Design review of the part built by this model. Coordinates are the model's own, in mm. Face numbers are marked on the shaded views. A direction names the side the tool comes from. Coordinates: 2 decimals unless noted, no trailing zeros. Write each loop counter-clockwise with the first axis right and the second up, starting at its lowest first coordinate (ties: lowest second). Pieces come first, ordered by that corner, then holes. Notation, with made-up numbers: (31.25, 24.25) -> (47.25, 24.25) arc R32 cw to (47.25, 62.25) -> close; hole circle Ø4 at (66, -30.75). An arc over 180 degrees is marked (long way). Answer in a Markdown table with one row per item. Add a question column.
Item 1: To check wall thickness, follow line 1 (Z direction, x = 0, y = 4); line 2 (X direction, y = 4, z = 2.5). State the ranges of each line that lie inside material, in increasing order.
Item 2: Take a section at B-B, the plane z = 0. Write out the cut boundary in (x, y).
Item 3: For the marked faces 4 and 5, list the 3-axis set-ups (+Z, -Z, +X, -X, +Y, -Y) from which the entire face can be reached by the end or side of a thin tool; tool diameter is ignored.
Item 4: Take a section at A-A, the plane x = 0. Write out the cut boundary in (y, z), and give its area (3 significant figures).
Item 5: Draft analysis for pull direction Z (two halves, no side actions). For the marked faces 1, 2 and 3, state which applies: released by +Z, released by -Z, zero draft, split by the parting line, or undercut.
Item 6: Clearance check with flat-ended pins moving along their axes: P1, Ø0.7, axis at x = 5.5, y = 0.5, coming from the +Z side; P2, Ø1, axis at y = 1.5, z = 5.5, coming from the +X side; P3, Ø0.7, axis at x = -4, y = 0.5, coming from the -Z side. State where each tip first meets the part, or that it passes through.
from build123d import *

# Parameters (mm, degrees)
SKETCH1_R               = 7.9375
SKETCH1_R_2             = 4.25
BOSS_EXTRUDE1_DEPTH     = 6.35
CUT_EXTRUDE1_DEPTH      = 13.896910967
CUT_EXTRUDE1_DEPTH_BACK = 13.896910967
SKETCH2_W               = 7.62
SKETCH2_H               = 2.54
FILLET2_R               = 1.905
FILLET3_R               = 1.27


with BuildPart() as part:
    # Sketch1 → Boss-Extrude1 (new body)
    with BuildSketch(Plane(origin=(0, 0, 0), x_dir=(1, 0, 0), z_dir=(0, 1, 0))):
        with Locations(Location((0, 0, 0), (0, 0, 270))):
            Circle(SKETCH1_R)
        with Locations(Location((0, 0, 0), (0, 0, 270))):
            Circle(SKETCH1_R_2, mode=Mode.SUBTRACT)
    extrude(amount=BOSS_EXTRUDE1_DEPTH)

    # Sketch2 → Cut-Extrude1 (cut, two sides: drawn at the far end of the back side and taken through both)
    with BuildSketch(Plane(origin=(0, 0, 0), x_dir=(0, 0, -1), z_dir=(1, 0, 0)).offset(-CUT_EXTRUDE1_DEPTH_BACK)):
        with Locations((0, 1.27)):
            Rectangle(SKETCH2_W, SKETCH2_H)
    extrude(amount=CUT_EXTRUDE1_DEPTH + CUT_EXTRUDE1_DEPTH_BACK, mode=Mode.SUBTRACT)

    # Fillet2
    fillet2_edges = [part.edges().sort_by_distance(p)[0] for p in [
        (4.423253704, 2.54, 3.81),
        (-4.423253704, 2.54, 3.81),
        (4.423253704, 2.54, -3.81),
        (-4.423253704, 2.54, -3.81),
    ]]
    fillet(fillet2_edges, radius=FILLET2_R)

    # Fillet3
    fillet3_edges = [part.edges().sort_by_distance(p)[0] for p in [
        (0, 6.35, -7.9375),
    ]]
    fillet(fillet3_edges, radius=FILLET3_R)


solid = part.part
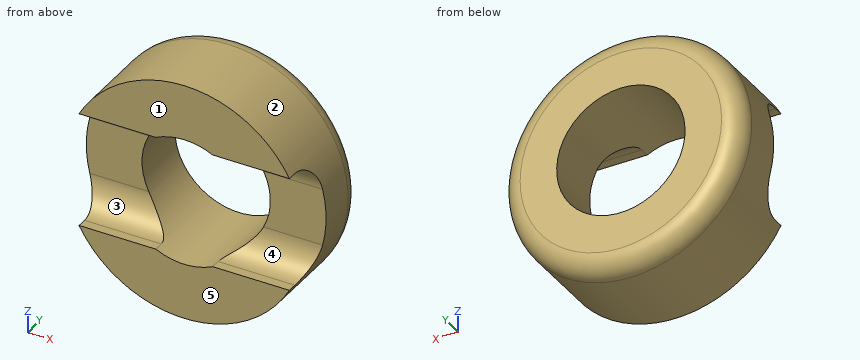
Answers:
| question | item | result |
|---|---|---|
| 1 | line 1 | z = -7.94 to -4.25, 4.25 to 7.94 |
| 1 | line 2 | x = -7.53 to -3.44, 3.44 to 7.53 |
| 2 | outline | (-7.94, 2.54) -> (-4.25, 2.54) -> (-4.25, 6.35) -> (-6.67, 6.35) arc R1.27 ccw to (-7.94, 5.08) -> close; (4.25, 2.54) -> (7.94, 2.54) -> (7.94, 5.08) arc R1.27 ccw to (6.67, 6.35) -> (4.25, 6.35) -> close |
| 3 | face 4 | +X, -X, -Y |
| 3 | face 5 | +Z, -Z, +X, -X, -Y |
| 4 | outline | (0, -7.94) -> (5.08, -7.94) arc R1.27 ccw to (6.35, -6.67) -> (6.35, -4.25) -> (0, -4.25) -> close; (0, 4.25) -> (6.35, 4.25) -> (6.35, 6.67) arc R1.27 ccw to (5.08, 7.94) -> (0, 7.94) -> close |
| 4 | area | 46.1 mm^2 |
| 5 | face 1 | zero draft |
| 5 | face 2 | split by the parting line |
| 5 | face 3 | undercut |
| 6 | P1 | stops at z = 6.04 |
| 6 | P2 | stops at x = 6.16 |
| 6 | P3 | stops at z = -7.05 |
